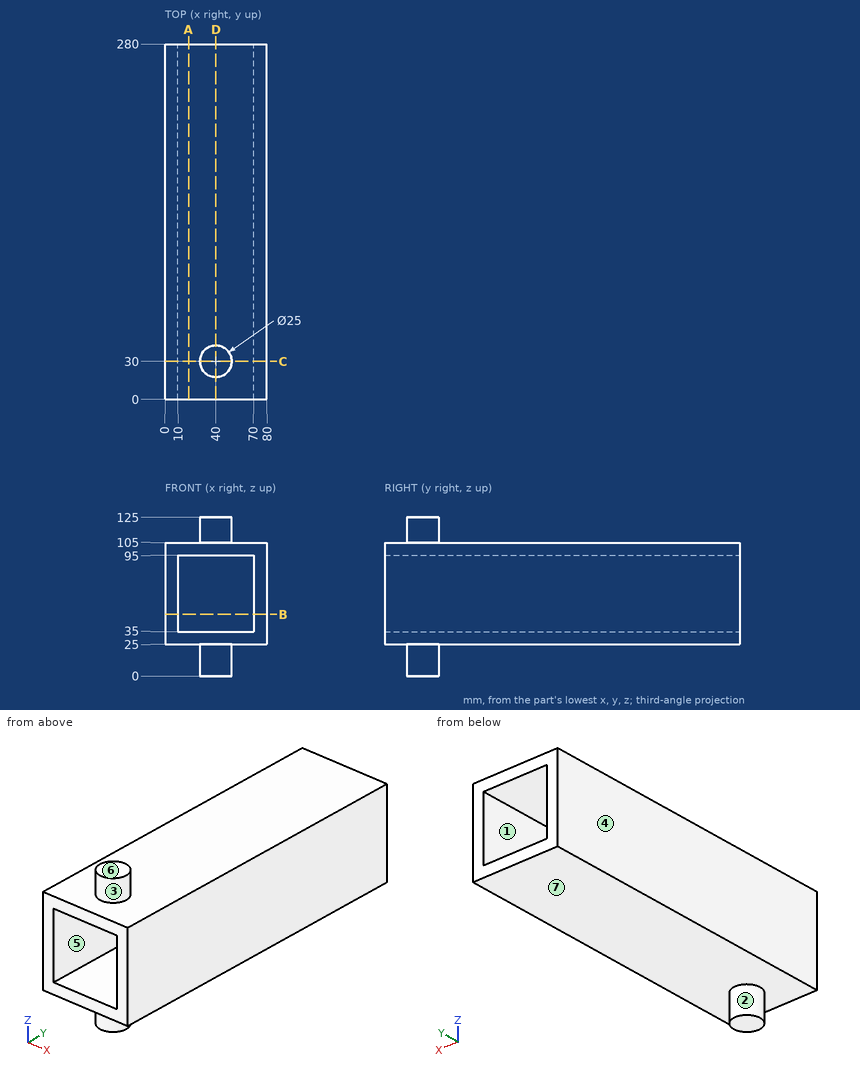
Geometry: see drawing. Coordinates: mm, zero at the bounding-box minimum. A direction names the side the tool comes from. Coordinates: 2 decimals unless noted, no trailing zeros. Loops run counter-clockwise (first coordinate to the right, second up) from the corner with the lowest first, then second, coordinate; pieces in that order, holes last.
(1) Section C-C on y = 30. Return the cut outline in (x, z), then the cut area to 4 significant figures.
(2) First-contact query: pin 1 Ø18 at (x, y) = (47.5, 100) entering from +Z; pin 2 Ø24 at (x, y) = (33, 196.5) entering from -Z; pin 3 Ø2 at (x, z) = (27.5, 14) entering from +Y. Flat tips, straight axial feed; report the tip coordinate or a pass-through.
(3) Section B-B on z = 48.5. Return the cut outline in (x, y).
(4) Set-up query: the marked faces 1, 2 and 3. Return all of +Z, -Z, +X, -X, +Y, -Y with unobstructed straight access to the full face (end or side cutting, diameter ignored); none if empty.
(5) Section A-A on x = 18.5. Return the cut outline in (y, z).
(6) Section D-D on x = 40. Return the cut outline in (y, z), then the cut area to 4 significant figures.
(7) Pull-direction query (Z, two-part tool) for the marked faces 4, 5, 6 and 7; classes: released by +Z, released by -Z, zero draft, split by the parting line, or undercut.
(8) Material intervals for probe 1 along X at (y, z) = (214, 37); probe 2 along Z at (x, y) = (47, 162.5); probe 3 along Z at (x, y) = (38.5, 24), sorted ascending.
Data:
1. outline: (0, 25) - (27.5, 25) - (27.5, 0) - (52.5, 0) - (52.5, 25) - (80, 25) - (80, 105) - (52.5, 105) - (52.5, 125) - (27.5, 125) - (27.5, 105) - (0, 105) - close; hole (10, 35) - (70, 35) - (70, 95) - (10, 95) - close
1. area: 3,925 mm2
2. pin 1: stops at z = 105
2. pin 2: stops at z = 25
2. pin 3: stops at y = 34.9
3. outline: (0, 0) - (10, 0) - (10, 280) - (0, 280) - close; (70, 0) - (80, 0) - (80, 280) - (70, 280) - close
4. face 1: +Y, -Y
4. face 2: -Z
4. face 3: +Z
5. outline: (0, 25) - (280, 25) - (280, 35) - (0, 35) - close; (0, 95) - (280, 95) - (280, 105) - (0, 105) - close
6. outline: (0, 25) - (17.5, 25) - (17.5, 0) - (42.5, 0) - (42.5, 25) - (280, 25) - (280, 35) - (0, 35) - close; (0, 95) - (280, 95) - (280, 105) - (42.5, 105) - (42.5, 125) - (17.5, 125) - (17.5, 105) - (0, 105) - close
6. area: 6,725 mm2
7. face 4: zero draft
7. face 5: undercut
7. face 6: released by +Z
7. face 7: released by -Z
8. probe 1: x = 0 to 10, 70 to 80
8. probe 2: z = 25 to 35, 95 to 105
8. probe 3: z = 0 to 35, 95 to 125
